Source: CAD feature listing. Evaluate the final solid. Frame: model axes, mm. Face numbers are marked on the shaded views. A direction names the side the tool comes from. Round coordinates to 2 decimals unless told otherwise and drop trailing zeros. Loops run counter-clockwise (first coordinate to the right, second up) from the corner with the lowest first, then second, coordinate; pieces in that order, holes last. Notation, with made-up numbers: M -2,-26.5 L 29,-26.5 A13 cw 29,-20.5 Z; hole C 66.25,58 d5. An arc over 180 degrees is marked long. Answer as a JSON object with one key per item and string values.
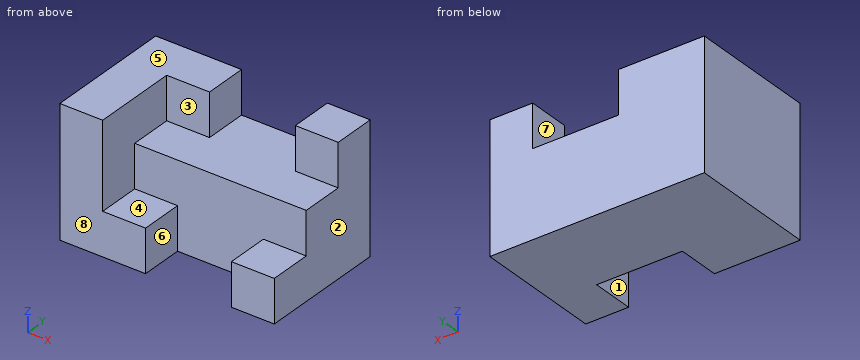
from build123d import *

# Parameters (mm, degrees)
F0_W     = 127
F0_H     = 76.2
F1_DEPTH = 76.2
F2_W     = 50.8
F2_H     = 25.4
F3_DEPTH = 86.868
F2_W_2   = 25.4
F4_DEPTH = 50.8
F5_DEPTH = 25.4


with BuildPart() as f1:
    # F0 (on Front) → F1 (new body)
    with BuildSketch(Plane.XZ):
        with Locations((15.835898, -27.176369)):
            Rectangle(F0_W, F0_H)
    extrude(amount=F1_DEPTH)

    # F2 (on face) → F3 (cut)
    with BuildSketch(Plane.XY.offset(10.923631)):
        with Locations((28.535898, -63.5)):
            Rectangle(F2_W, F2_H)
    extrude(amount=-F3_DEPTH, mode=Mode.SUBTRACT)

    # F2 (on face) → F4 (cut)
    with BuildSketch(Plane.XY.offset(10.923631)):
        with Locations((-9.564102, -63.5)):
            Rectangle(F2_W_2, F2_H)
        with Locations((66.635898, -63.5)):
            Rectangle(F2_W_2, F2_H)
    extrude(amount=-F4_DEPTH, mode=Mode.SUBTRACT)

    # F2 (on face) → F5 (cut)
    with BuildSketch(Plane.XY.offset(10.923631)):
        Polygon((53.935898, -25.4), (53.935898, 0), (3.135898, 0), (3.135898, -25.38896), (-22.264102, -25.38896), (-22.264102, -50.8), (3.135898, -50.8), (53.935898, -50.8), (79.335898, -50.8), (79.335898, -25.4), align=None)
    extrude(amount=-F5_DEPTH, mode=Mode.SUBTRACT)


solid = f1.part
Item 1: Section D-D on x = -20. Return the cut outline in (y, z), then the cut area to 3 significant figures.
Answer sheet:
{"outline": "M -76.2,-65.28 L 0,-65.28 L 0,10.92 L -25.39,10.92 L -25.39,-14.48 L -50.8,-14.48 L -50.8,-39.88 L -76.2,-39.88 Z", "area": "3,870 mm²"}
Item 2: Section B-B on z = -18. Return the cut outline in (x, y), then the cut area to 3 significant figures.
Answer sheet:
{"outline": "M -47.66,-76.2 L -22.26,-76.2 L -22.26,-50.8 L 79.34,-50.8 L 79.34,0 L -47.66,0 Z", "area": "7,100 mm²"}
Item 3: Section C-C on y = -15. Return the cut outline in (x, z).
Answer sheet:
{"outline": "M -47.66,-65.28 L 79.34,-65.28 L 79.34,10.92 L 53.94,10.92 L 53.94,-14.48 L 3.14,-14.48 L 3.14,10.92 L -47.66,10.92 Z"}
Item 4: Pull-direction query (X, two-part tool) for the marked faces 1, 2 and 3; classes: pulls with the +X half, pulls with the -X half, needs draft (parallel to the pull), parting line crosses it, or undercut.
Answer sheet:
{"face 1": "undercut", "face 2": "pulls with the +X half", "face 3": "needs draft"}
Item 5: Access query for the marked faces 4, 5, 6, 7 and 8. Directions: +Z, -Z, +X, -X, +Y, -Y. A direction counts if a zero-diameter tool reaches every point of the face in a straight line with its end or side. Return the directions, or none.
Answer sheet:
{"face 4": "+Z, +X, -Y", "face 5": "+Z, +X, -X, +Y, -Y", "face 6": "+Z, -Z, -Y", "face 7": "+Z, +Y, -Y", "face 8": "+Z, -Z, +X, -X, -Y"}
Item 6: Line query: probe 1 along X at (y, z) = (-14.5, -4.5); probe 2 along Z at (x, y) = (-0.5, -58.5); probe 3 along Z at (x, y) = (71, -47). Output: solid intervals per line, ascending. Write a range as from..to.
Answer sheet:
{"probe 1": "x = -47.66..3.14, 53.94..79.34", "probe 2": "z = -65.28..-39.88", "probe 3": "z = -65.28..-14.48"}
Item 7: Section A-A on y = -56. Return the cut outline in (x, z).
Answer sheet:
{"outline": "M -47.66,-65.28 L 3.14,-65.28 L 3.14,-39.88 L -22.26,-39.88 L -22.26,10.92 L -47.66,10.92 Z; M 53.94,-65.28 L 79.34,-65.28 L 79.34,-39.88 L 53.94,-39.88 Z"}
Item 8: Contact query for flat-ended pins moving along their axis: pin 1 Ø1.5 at (y, z) = (-38, -1.5) entering from +X; pin 2 Ø4 at (x, y) = (19, -43.5) entering from +Z; pin 3 Ø7.5 at (x, y) = (-7.5, -60.5) entering from +Z. Output: stop coordinate, or through.
Answer sheet:
{"pin 1": "stops at x = -22.26", "pin 2": "stops at z = -14.48", "pin 3": "stops at z = -39.88"}
